Geometry check sheet. Reference: the model listing, model coordinates, mm. Face numbers are marked on the shaded views. A direction names the side the tool comes from. Round coordinates to 2 decimals unless told otherwise and drop trailing zeros. Write each loop counter-clockwise with the first axis right and the second up, starting at its lowest first coordinate (ties: lowest second). Pieces come first, ordered by that corner, then holes.
Item 1: Depth check by flat-ended pin: P1, Ø3, axis at x = 8, y = -32, coming from the +Z side; P2, Ø4, axis at y = -21, z = 4, coming from the -X side; P3, Ø6.5, axis at y = -34.5, z = 8.5, coming from the +X side. Enter the tip coordinate at first touch or a pass-through.
Item 2: Cross-section at A-A (z = 8.75). Enter the section's corners in (x, y).
Item 3: Cross-section at B-B (y = -34). Enter the section's corners in (x, z).
Item 4: Cross-section at C-C (x = 9). Enter the section's corners in (y, z), then the cut area to 3 significant figures.
Item 5: Access from +Z, -Z, +X, -X, +Y, -Y to the whole of each face (thin tool, end or side, straight path). Record for the marked faces 1 and 2.
Item 6: Scan lines: probe 1 along X at (y, z) = (-20.5, 10.5); probe 2 along Z at (x, y) = (-10.25, -31); probe 3 along Y at (x, z) = (-8.75, 8.75). Record each from-to range of solid material in increasing order.
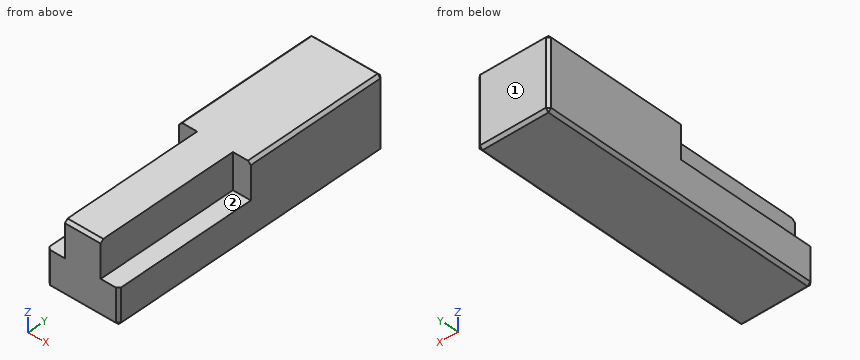
from build123d import *

# Parameters (mm, degrees)
F0_W     = 25.4
F0_H     = 25.4
F1_DEPTH = 50.8
F2_W     = 6.35
F2_H     = 12.7
F3_DEPTH = 50.8
F4_SIZE  = 1


with BuildPart() as f1:
    # F0 (on Front) → F1 (new body, symmetric)
    with BuildSketch(Plane.XZ):
        Rectangle(F0_W, F0_H)
    extrude(amount=F1_DEPTH, both=True)

    # F2 (on face) → F3 (cut)
    with BuildSketch(Plane.XZ.offset(50.8)):
        with Locations((-9.525, 6.35)):
            Rectangle(F2_W, F2_H)
        with Locations((9.525, 6.35)):
            Rectangle(F2_W, F2_H)
    extrude(amount=-F3_DEPTH, mode=Mode.SUBTRACT)

    # F4
    f4_edges = [f1.edges().sort_by_distance(p)[0] for p in [
        (12.7, 25.4, 12.7),
        (12.7, 0, -12.7),
        (12.7, 50.8, 0),
        (12.7, -50.8, -6.35),
        (0, -50.8, 12.7),
        (-12.7, -50.8, -6.35),
        (-12.7, 25.4, 12.7),
        (0, 50.8, 12.7),
        (0, -50.8, -12.7),
        (-12.7, 0, -12.7),
        (-12.7, 50.8, 0),
        (0, 50.8, -12.7),
    ]]
    chamfer(f4_edges, length=F4_SIZE)


solid = f1.part
Resolved:
1. P1: stops at z = 0
1. P2: stops at x = -6.35
1. P3: stops at x = 6.35
2. outline: (-12.7, 0) - (-6.35, 0) - (-6.35, -50.8) - (6.35, -50.8) - (6.35, 0) - (12.7, 0) - (12.7, 49.8) - (11.7, 50.8) - (-11.7, 50.8) - (-12.7, 49.8) - close
3. outline: (-12.7, -11.7) - (-11.7, -12.7) - (11.7, -12.7) - (12.7, -11.7) - (12.7, 0) - (6.35, 0) - (6.35, 12.7) - (-6.35, 12.7) - (-6.35, 0) - (-12.7, 0) - close
4. outline: (-50.8, -11.7) - (-49.8, -12.7) - (49.8, -12.7) - (50.8, -11.7) - (50.8, 11.7) - (49.8, 12.7) - (0, 12.7) - (0, 0) - (-50.8, 0) - close
4. area: 1,930 mm2
5. face 1: +Z, -Z, +X, -X, +Y
5. face 2: +Z, +X, -Y
6. probe 1: x = -6.35 to 6.35
6. probe 2: z = -12.7 to 0
6. probe 3: y = 0 to 50.8
